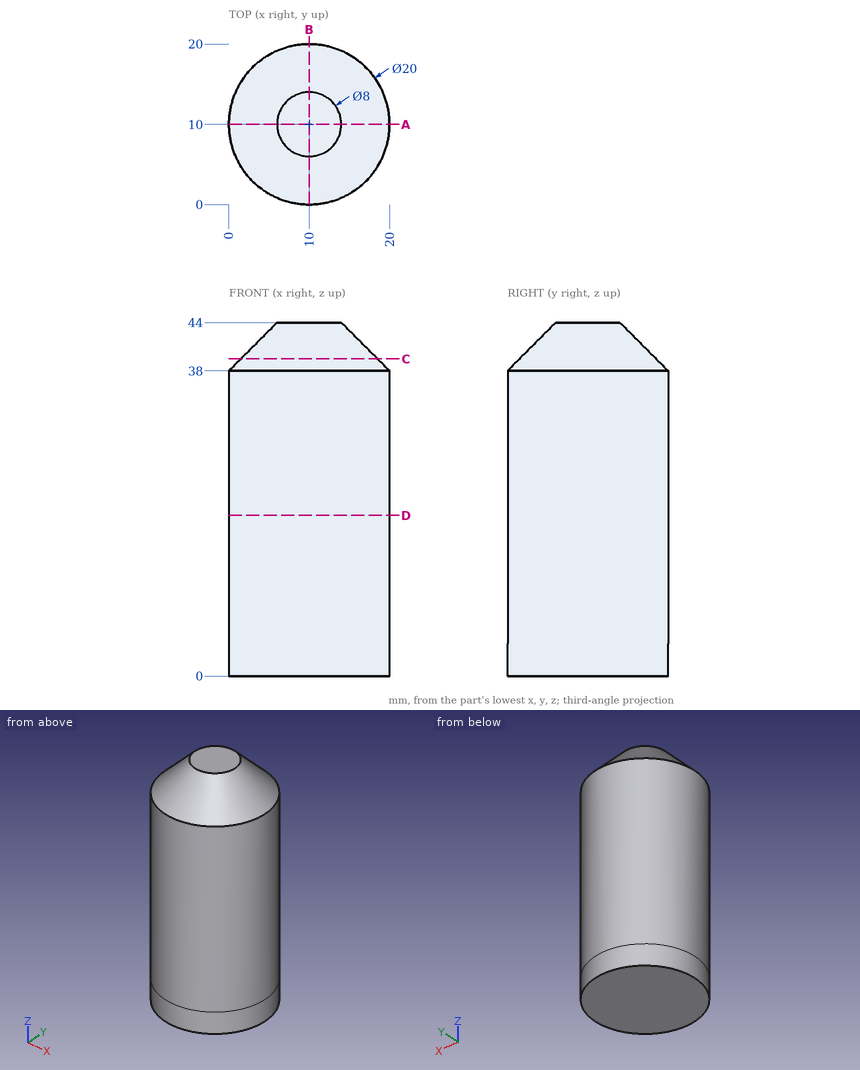
Design review of the part shown in the three views and the two pictorial views. Dimensions are in mm from the part's minimum x, y and z. Round coordinates to 2 decimals unless told otherwise and drop trailing zeros. Write each loop counter-clockwise with the first axis right and the second up, starting at its lowest first coordinate (ties: lowest second). Pieces come first, ordered by that corner, then holes. Notation, with made-up numbers: (-13, 30) - (-3, 30) arc R7 ccw to (-3, 34) - close; hole circle Ø4 at (25, -12). An arc over 180 degrees is marked (long way). Write item = value, one per line. Start each with the question number.
1. Consider section C-C on z = 39.5. State the section outline as (x, y) points, plus the area to 3 significant figures.
2. Consider section D-D on z = 20. State the section outline as (x, y) points.
3. Wall thickness on L1, parallel to Y at x = 10, z = 18.5; L2, parallel to X at y = 6, z = 31.5; L3, parallel to Z at x = 8.5, y = 3.75: over which ranges is each line inside the solid? List them lowest first.
4. For pin 1 Ø1 at (x, y) = (9.5, 2) entering from +Z; pin 2 Ø1 at (y, z) = (12, 18.5) entering from -X; pin 3 Ø4 at (x, z) = (5.5, 26) entering from -Y, all flat-tipped, find the tip position at first contact; note any pin that passes through.
5. Consider section A-A on y = 10. State the section outline as (x, z) points.
Evaluation:
q1.outline = circle Ø17 at (10, 10)
q1.area = 227 mm2
q2.outline = circle Ø20 at (10, 10)
q3.L1 = 0 to 20
q3.L2 = 0.83 to 19.17
q3.L3 = 0 to 41.57
q4.pin_1 = 40.48
q4.pin_2 = 0.11
q4.pin_3 = 0.32
q5.outline = (0, 0) - (20, 0) - (20, 38) - (14, 44) - (6, 44) - (0, 38) - close
